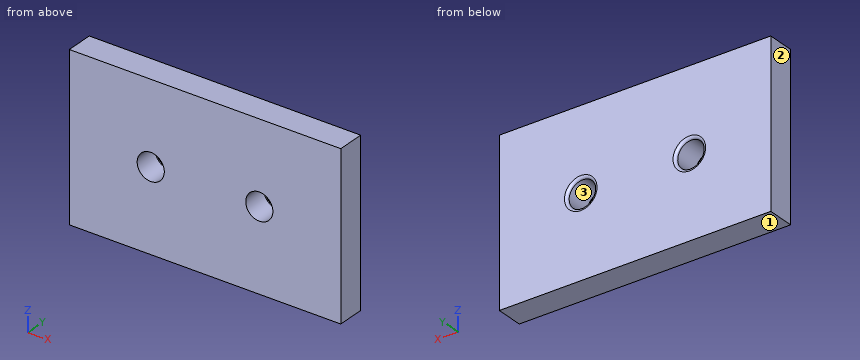
```python
from build123d import *

# Parameters (mm, degrees)
SKETCH_1_W          = 100
SKETCH_1_H          = 60
EXTRUDE_1_DEPTH     = 10
SKETCH_2_R          = 5
CUT_EXTRUDE_1_DEPTH = 20
SKETCH_3_R          = 5
CUT_EXTRUDE_2_DEPTH = 20
FILLET_1_R          = 1


with BuildPart() as part:
    # 草图1 → 凸台-拉伸1 (new body)
    with BuildSketch(Plane(origin=(0, 0, 0), x_dir=(1, 0, 0), z_dir=(0, 1, 0))):
        Rectangle(SKETCH_1_W, SKETCH_1_H)
    extrude(amount=EXTRUDE_1_DEPTH)

    # 草图2 → 切除-拉伸1 (cut)
    with BuildSketch(Plane(origin=(0, 0, 0), x_dir=(1, 0, 0), z_dir=(0, 1, 0))):
        with Locations(Location((-20, 0, 0), (0, 0, 90))):
            Circle(SKETCH_2_R)
    extrude(amount=CUT_EXTRUDE_1_DEPTH, mode=Mode.SUBTRACT)

    # 草图3 → 切除-拉伸2 (cut)
    with BuildSketch(Plane(origin=(0, 0, 0), x_dir=(1, 0, 0), z_dir=(0, 1, 0))):
        with Locations(Location((20, 0, 0), (0, 0, 90))):
            Circle(SKETCH_3_R)
    extrude(amount=CUT_EXTRUDE_2_DEPTH, mode=Mode.SUBTRACT)

    # 圆角1
    fillet_1_edges = [part.edges().sort_by_distance(p)[0] for p in [
        (-20, 10, 5),
        (20, 10, 5),
    ]]
    fillet(fillet_1_edges, radius=FILLET_1_R)


solid = part.part
```
Geometry check sheet. Reference: the model listing, model coordinates, mm. Face numbers are marked on the shaded views. Give positions to 0.01 mm unless a question says otherwise; leave off trailing zeros. Order: outer loops, then holes, each group sorted by start corner. A loop starts at its lowest first (then second) coordinate and runs counter-clockwise, first axis right, second up. Notation, with made-up numbers: (-39, 74.25) - (-8, 74.25) arc R14 cw to (-8, 80.25) - close; hole circle Ø8 at (85, -3). An arc over 180 degrees is marked (long way). Write item = value, one per line. Start each with the question number.
1) Draft check along Z on the marked faces 1, 2 and 3. Enter one of: released by +Z, released by -Z, zero draft, split by the parting line, or undercut.
2) Gauge pin test, flat ends, axial feed: pin 1 Ø4 at (x, z) = (-37.5, 18) entering from -Y; pin 2 Ø9 at (x, z) = (-20, 0) entering from -Y. Record the tip position at first contact, or that the pin passes through.
3) Section check C-C (y = 6.25). Enter the section's corners in (x, z).
4) Section check A-A (x = 20). Enter the section's corners in (y, z).
5) Scan lines: L1, parallel to X at y = 2.5, z = 0; L2, parallel to Z at x = 20, y = 7.25; L3, parallel to X at y = 8.5, z = 3.5. Record each from-to range of solid material in increasing order.
6) Section check B-B (z = 0). Enter the section's corners in (x, y).
Geometry check:
q1.face_1 = released by -Z
q1.face_2 = zero draft
q1.face_3 = undercut
q2.pin_1 = 0
q2.pin_2 = through
q3.outline = (-50, -30) - (50, -30) - (50, 30) - (-50, 30) - close; hole circle Ø10 at (-20, 0); hole circle Ø10 at (20, 0)
q4.outline = (0, -30) - (10, -30) - (10, -6) arc R1 ccw to (9, -5) - (0, -5) - close; (0, 5) - (9, 5) arc R1 ccw to (10, 6) - (10, 30) - (0, 30) - close
q5.L1 = -50 to -25, -15 to 15, 25 to 50
q5.L2 = -30 to -5, 5 to 30
q5.L3 = -50 to -23.57, -16.43 to 16.43, 23.57 to 50
q6.outline = (-50, 0) - (-25, 0) - (-25, 9) arc R1 ccw to (-26, 10) - (-50, 10) - close; (-15, 0) - (15, 0) - (15, 9) arc R1 ccw to (14, 10) - (-14, 10) arc R1 ccw to (-15, 9) - close; (25, 0) - (50, 0) - (50, 10) - (26, 10) arc R1 ccw to (25, 9) - close
